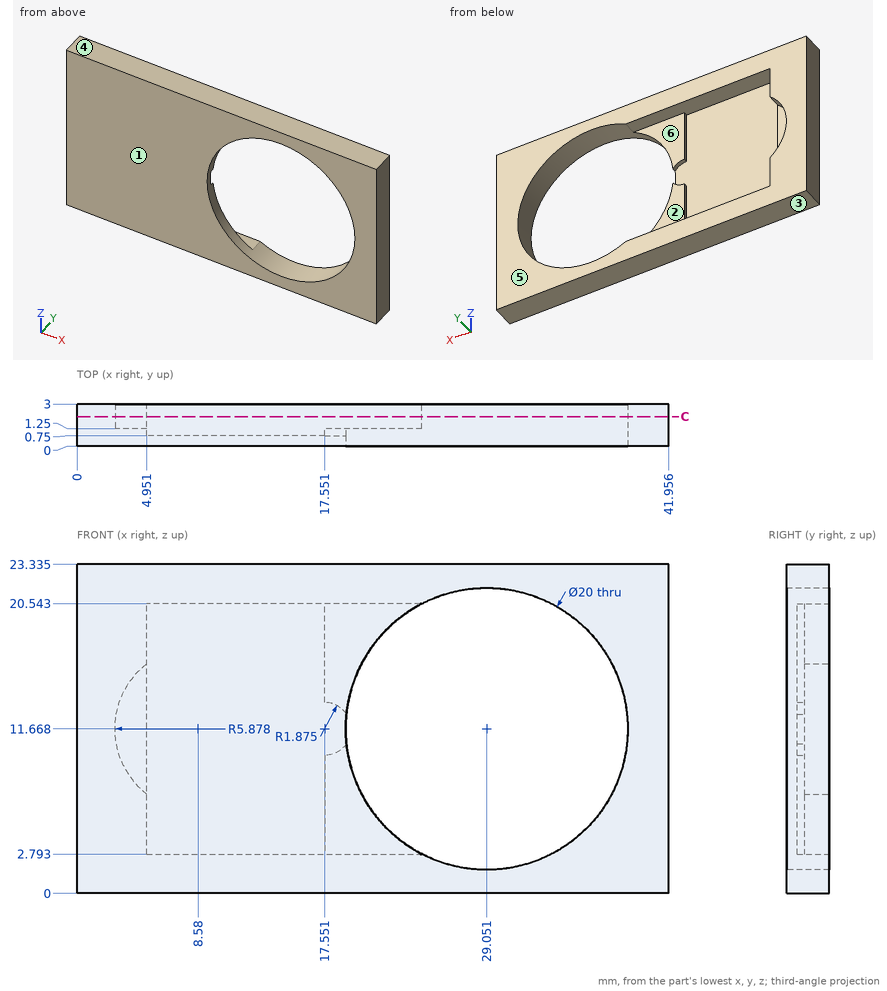
Print and shaded views of the part. All mm, measured from the part's lowest x, y and z. A direction names the side the tool comes from. Coordinates: 2 decimals unless noted, no trailing zeros. Write each loop counter-clockwise with the first axis right and the second up, starting at its lowest first coordinate (ties: lowest second). Pieces come first, ordered by that corner, then holes. Notation, with made-up numbers: (0.5, -29.75) -> (4.5, -29.75) arc R21 ccw to (4.5, -0.75) -> close; hole circle Ø9 at (77.25, 4). An arc over 180 degrees is marked (long way). Use CSV: the item, a comma, the result in double quotes. Start each with the question number.
Q1. Pull direction Z, two halves, no side cores. Call the marked faces 1, 2, 3 and 4: released by +Z, released by -Z, zero draft, split by the parting line, or undercut.
Q2. Flat gauge pins, fed straight in: pin 1 Ø8 at (x, z) = (9, 16.5) entering from +Y; pin 2 Ø0.7 at (x, z) = (4, 13) entering from +Y. Where does each tip first touch, or does it go through?
Q3. Cut at C-C, the plane y = 2.1. List the corners of the cut face in (x, z) (1 decimal).
Q4. 3-axis set-ups, long thin cutter, end or side, ignore diameter. For the marked faces 5 and 6: which of +Z, -Z, +X, -X, +Y, -Y reach the whole face in a straight line?
Q5. Drill centre lines: probe 1 along Z at (x, y) = (21.5, 2.25) (1 decimal); probe 2 along Y at (x, z) = (4, 10.5); probe 3 along Y at (x, z) = (6.5, 14.5). Where is each one in solid material? Low to high.
Checked values:
1,face 1,"zero draft"
1,face 2,"undercut"
1,face 3,"released by -Z"
1,face 4,"released by +Z"
2,pin 1,"stops at y = 0.75"
2,pin 2,"stops at y = 1.25"
3,outline,"(0, 0) -> (42, 0) -> (42, 23.3) -> (0, 23.3) -> close; hole (5, 2.8) -> (24.4, 2.8) arc R10 ccw (long way) to (24.4, 20.5) -> (5, 20.5) -> (5, 16.3) arc R5.9 ccw to (5, 7) -> close"
4,face 5,"+Z, -Z, +X, -X, +Y"
4,face 6,"+Y"
5,probe 1,"z = 0 to 2.8, 20.5 to 23.3"
5,probe 2,"y = 0 to 1.25"
5,probe 3,"y = 0 to 0.75"
